Verification items for the finished model (mm, model axes). Give positions to 0.01 mm unless a question says otherwise; leave off trailing zeros. Loops run counter-clockwise (first coordinate to the right, second up) from the corner with the lowest first, then second, coordinate; pieces in that order, holes last. Notation, with made-up numbers: (36, 14) - (54, 14) arc R16 ccw to (54, 32) - close; hole circle Ø3 at (42, 56). An arc over 180 degrees is marked (long way). One line per item, written item: value. Start each with the question number.
1. Sectioned sample at B-B (z = 4.75). Count the separate pieces of the cut face and the enclosed holes in it, plus the area to 3 significant figures.
2. Sectioned sample at A-A (x = 247.65). Record the cut outline in (y, z).
3. Gauge pin test, flat end, axial feed: pin 1 (7.5 mm diameter, centred on x = 304.55, y = -48.59, fed in from +Z). Record the tip position at first contact, or that the pin passes through.
4. Scan lines: L1, parallel to Y at x = 105.41, z = 2.25; L2, parallel to Y at x = 21.5, z = 4; L3, parallel to X at y = -4, z = 4.75 (3 decimals). Record each from-to range of solid material in increasing order. Write a range as [from, to].
from build123d import *

# Parameters (mm, degrees)
F0_R     = 6.35
F1_DEPTH = 6.35


with BuildPart() as f1:
    # F0 (on Top) → F1 (new body)
    with BuildSketch(Plane.XY):
        with BuildLine():
            Line((76.2, 0), (6.35, 0))
            ThreePointArc((6.35, 0), (1.859872, -1.859872), (0, -6.35))
            Line((0, -6.35), (0, -57.15))
            ThreePointArc((0, -57.15), (1.859872, -61.640128), (6.35, -63.5))
            Line((6.35, -63.5), (488.95, -63.5))
            ThreePointArc((488.95, -63.5), (493.440128, -61.640128), (495.3, -57.15))
            Line((495.3, -57.15), (495.3, -6.35))
            ThreePointArc((495.3, -6.35), (493.440128, -1.859872), (488.95, 0))
            Line((488.95, 0), (419.1, 0))
            Line((419.1, 0), (419.1, -5.08))
            Line((419.1, -5.08), (361.95, -5.08))
            Line((361.95, -5.08), (361.95, 0))
            Line((361.95, 0), (276.225, 0))
            Line((276.225, 0), (276.225, -5.08))
            Line((276.225, -5.08), (219.075, -5.08))
            Line((219.075, -5.08), (219.075, 0))
            Line((219.075, 0), (133.35, 0))
            Line((133.35, 0), (133.35, -5.08))
            Line((133.35, -5.08), (76.2, -5.08))
            Line((76.2, -5.08), (76.2, 0))
        make_face()
        with Locations((20.066, -48.587607)):
            Circle(F0_R, mode=Mode.SUBTRACT)
        with Locations((48.514, -48.587607)):
            Circle(F0_R, mode=Mode.SUBTRACT)
        with Locations((76.962, -48.587607)):
            Circle(F0_R, mode=Mode.SUBTRACT)
        with Locations((105.41, -48.587607)):
            Circle(F0_R, mode=Mode.SUBTRACT)
        with Locations((133.858, -48.587607)):
            Circle(F0_R, mode=Mode.SUBTRACT)
        with Locations((162.306, -48.587607)):
            Circle(F0_R, mode=Mode.SUBTRACT)
        with Locations((190.754, -48.587607)):
            Circle(F0_R, mode=Mode.SUBTRACT)
        with Locations((219.202, -48.587607)):
            Circle(F0_R, mode=Mode.SUBTRACT)
        with Locations((247.65, -48.587607)):
            Circle(F0_R, mode=Mode.SUBTRACT)
        with Locations((276.098, -48.587607)):
            Circle(F0_R, mode=Mode.SUBTRACT)
        with Locations((304.546, -48.587607)):
            Circle(F0_R, mode=Mode.SUBTRACT)
        with Locations((332.994, -48.587607)):
            Circle(F0_R, mode=Mode.SUBTRACT)
        with Locations((361.442, -48.587607)):
            Circle(F0_R, mode=Mode.SUBTRACT)
        with Locations((389.89, -48.587607)):
            Circle(F0_R, mode=Mode.SUBTRACT)
        with Locations((418.338, -48.587607)):
            Circle(F0_R, mode=Mode.SUBTRACT)
        with Locations((446.786, -48.587607)):
            Circle(F0_R, mode=Mode.SUBTRACT)
        with Locations((475.234, -48.587607)):
            Circle(F0_R, mode=Mode.SUBTRACT)
        with Locations((20.066, -21.238256)):
            Circle(F0_R, mode=Mode.SUBTRACT)
        with Locations((48.514, -21.238256)):
            Circle(F0_R, mode=Mode.SUBTRACT)
        with Locations((76.962, -21.238256)):
            Circle(F0_R, mode=Mode.SUBTRACT)
        with Locations((105.41, -21.238256)):
            Circle(F0_R, mode=Mode.SUBTRACT)
        with Locations((133.858, -21.238256)):
            Circle(F0_R, mode=Mode.SUBTRACT)
        with Locations((162.306, -21.238256)):
            Circle(F0_R, mode=Mode.SUBTRACT)
        with Locations((190.754, -21.238256)):
            Circle(F0_R, mode=Mode.SUBTRACT)
        with Locations((219.202, -21.238256)):
            Circle(F0_R, mode=Mode.SUBTRACT)
        with Locations((247.65, -21.238256)):
            Circle(F0_R, mode=Mode.SUBTRACT)
        with Locations((276.098, -21.238256)):
            Circle(F0_R, mode=Mode.SUBTRACT)
        with Locations((304.546, -21.238256)):
            Circle(F0_R, mode=Mode.SUBTRACT)
        with Locations((332.994, -21.238256)):
            Circle(F0_R, mode=Mode.SUBTRACT)
        with Locations((361.442, -21.238256)):
            Circle(F0_R, mode=Mode.SUBTRACT)
        with Locations((389.89, -21.238256)):
            Circle(F0_R, mode=Mode.SUBTRACT)
        with Locations((418.338, -21.238256)):
            Circle(F0_R, mode=Mode.SUBTRACT)
        with Locations((446.786, -21.238256)):
            Circle(F0_R, mode=Mode.SUBTRACT)
        with Locations((475.234, -21.238256)):
            Circle(F0_R, mode=Mode.SUBTRACT)
    extrude(amount=F1_DEPTH)


solid = f1.part
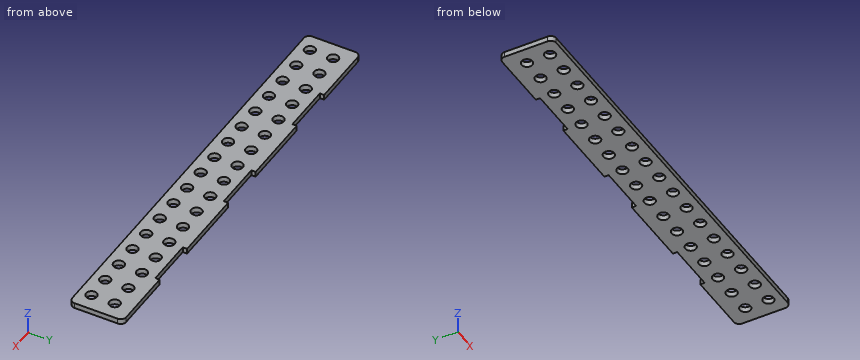
Results are:
1. separate pieces: 1
1. enclosed holes: 34
1. area: 26,200 mm^2
2. outline: (-63.5, 0) - (-54.94, 0) - (-54.94, 6.35) - (-63.5, 6.35) - close; (-42.24, 0) - (-27.59, 0) - (-27.59, 6.35) - (-42.24, 6.35) - close; (-14.89, 0) - (-5.08, 0) - (-5.08, 6.35) - (-14.89, 6.35) - close
3. pin 1: passes through
4. L1: y = [-63.5, -54.94], [-42.24, -27.59], [-14.89, -5.08]
4. L2: y = [-63.5, -54.77], [-42.4, -27.42], [-15.05, 0]
4. L3: x = [0.451, 76.2], [133.35, 219.075], [276.225, 361.95], [419.1, 494.849]
